Read the model definition and answer for the solid it produces. Units are mm, in the model's axes. Coordinates: 2 decimals unless noted, no trailing zeros. Order: outer loops, then holes, each group sorted by start corner. A loop starts at its lowest first (then second) coordinate and runs counter-clockwise, first axis right, second up. Notation, with made-up numbers: M 43.25,-19 L 96.25,-19 A32 cw 96.25,9 Z; hole C 34.25,-12.5 d2. An arc over 180 degrees is marked long. Use a Markdown table: item, result. Add a question column.
1) Find section A-A on x = -12.5. Write down the section's boundary in (y, z), plus the area to 3 significant figures.
2) Find section B-B on z = -120. Write down the section's boundary in (x, y), plus the area to 3 significant figures.
3) Find the intervals of material crossed by probe 1 along Z at (x, y) = (-135, -2.55); probe 2 along X at (y, z) = (-0.2, -120), in increasing order. Write a range as [from, to].
4) This flat-tipped pin is pushed along its axis until it touches: pin 1 Ø3 at (x, z) = (135, 135) entering from -Y. Where does it stop, or does it pass through?
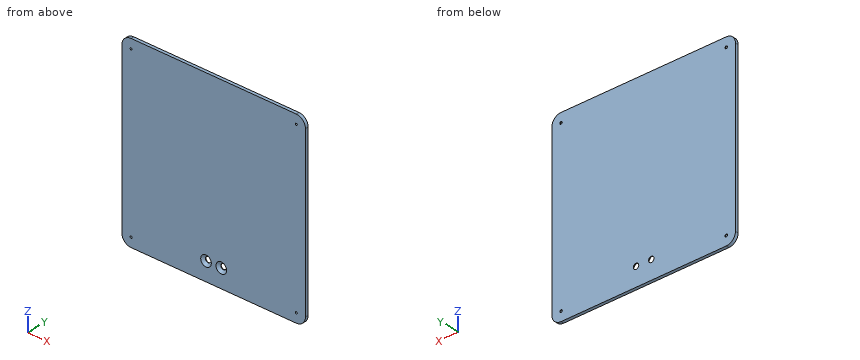
from build123d import *

# Parameters (mm, degrees)
ESQUISSE1_W                                 = 300
ESQUISSE1_H                                 = 300
T_LE_DE_BASE_PLI_E1_DEPTH                   = 5
FRAISAGE_POUR_VIS_T_TE_FRAIS_E_M81_AT_COUNT = 2
FRAISAGE_POUR_VIS_T_TE_FRAIS_E_M81_AT_PITCH = 25
TROU_TARAUD_M41_D                           = 3.3
TROU_TARAUD_M41_CSINK_D                     = 4.05
TROU_TARAUD_M41_CSINK_ANGLE                 = 90
CONG_1_R                                    = 15


# Sheet-metal steps are written as plain solids
with BuildPart() as part:
    # Esquisse1 → Tôle de base pliée1 (new body)
    with BuildSketch(Plane(origin=(0, 0, 0), x_dir=(1, 0, 0), z_dir=(0, 1, 0))):
        Rectangle(ESQUISSE1_W, ESQUISSE1_H)
    extrude(amount=-T_LE_DE_BASE_PLI_E1_DEPTH)

    # Esquisse3 → Fraisage pour vis à tête fraisée M81 (revolve, cut)
    with BuildSketch(Plane(origin=(12.5, -5, -120), x_dir=(0, 0, -1), z_dir=(1, 0, 0))):
        Polygon((0, 0), (0, 5), (4.5, 5), (4.5, 4.15), (8.65, 0), align=None)
    fraisage_pour_vis_t_te_frais_e_m81 = revolve(axis=Axis((12.5, -11.35, -120), (0, 1, 0)), mode=Mode.SUBTRACT)

    # Fraisage pour vis à tête fraisée M81 at: Fraisage pour vis à tête fraisée M81 ×2
    with Locations(*[(-i * FRAISAGE_POUR_VIS_T_TE_FRAIS_E_M81_AT_PITCH, 0, 0) for i in range(1, FRAISAGE_POUR_VIS_T_TE_FRAIS_E_M81_AT_COUNT)]):
        add(fraisage_pour_vis_t_te_frais_e_m81, mode=Mode.SUBTRACT)

    # Trou taraudé M41 (through all)
    with Locations(Plane(origin=(0, 0, 0), x_dir=(1, 0, 0), z_dir=(0, 1, 0))):
        with Locations((135, -135), (-135, -135), (-135, 135), (135, 135)):
            CounterSinkHole(TROU_TARAUD_M41_D / 2, TROU_TARAUD_M41_CSINK_D / 2, counter_sink_angle=TROU_TARAUD_M41_CSINK_ANGLE)

    # Congé1
    cong_1_edges = [part.edges().sort_by_distance(p)[0] for p in [
        (-150, -2.5, -150),
        (150, -2.5, -150),
        (150, -2.5, 150),
        (-150, -2.5, 150),
    ]]
    fillet(cong_1_edges, radius=CONG_1_R)


solid = part.part
Check result:
| question | item | result |
|---|---|---|
| 1 | outline | M -5,-150 L 0,-150 L 0,-124.5 L -0.85,-124.5 L -5,-128.65 Z; M -5,-111.35 L -0.85,-115.5 L 0,-115.5 L 0,150 L -5,150 Z |
| 1 | area | 1,440 mm2 |
| 2 | outline | M -150,-5 L -21.15,-5 L -17,-0.85 L -17,0 L -150,0 Z; M -8,-0.85 L -3.85,-5 L 3.85,-5 L 8,-0.85 L 8,0 L -8,0 Z; M 17,-0.85 L 21.15,-5 L 150,-5 L 150,0 L 17,0 Z |
| 2 | area | 1,380 mm2 |
| 3 | probe 1 | z = [-150, -136.65], [-133.35, 133.35], [136.65, 150] |
| 3 | probe 2 | x = [-150, -17], [-8, 8], [17, 150] |
| 4 | pin 1 | passes through |
